Read the model definition and answer for the solid it produces. Units are mm, in the model's axes. Coordinates: 2 decimals unless noted, no trailing zeros. Order: outer loops, then holes, each group sorted by start corner. A loop starts at its lowest first (then second) coordinate and runs counter-clockwise, first axis right, second up.
```python
from build123d import *

# Parameters (mm, degrees)
SKETCH_W   = 80
SKETCH_H   = 120
SKETCH_R   = 4.5
SKETCH_R_2 = 11
SKETCH_R_3 = 3
PAD_DEPTH  = 10


with BuildPart() as part:
    # Sketch → Pad (new body)
    with BuildSketch(Plane.XY):
        with Locations((15, -15)):
            Rectangle(SKETCH_W, SKETCH_H)
        Circle(SKETCH_R, mode=Mode.SUBTRACT)
        with Locations((0, -30)):
            Circle(SKETCH_R_2, mode=Mode.SUBTRACT)
        with Locations((-10, -52)):
            Circle(SKETCH_R_3, mode=Mode.SUBTRACT)
        with Locations((40, -52)):
            Circle(SKETCH_R_3, mode=Mode.SUBTRACT)
        with Locations((40, 22)):
            Circle(SKETCH_R_3, mode=Mode.SUBTRACT)
        with Locations((-10, 22)):
            Circle(SKETCH_R_3, mode=Mode.SUBTRACT)
    extrude(amount=PAD_DEPTH)


solid = part.part
```
1) A cutting plane is placed at B-B, the plane y = -52. Determine the outline of the cut face in (x, z).
A:
outline: (-25, 0) - (-13, 0) - (-13, 10) - (-25, 10) - close; (-7, 0) - (37, 0) - (37, 10) - (-7, 10) - close; (43, 0) - (55, 0) - (55, 10) - (43, 10) - close
2) A cutting plane is placed at C-C, the plane z = 5. Determine the outline of the cut face in (x, y).
A:
outline: (-25, -75) - (55, -75) - (55, 45) - (-25, 45) - close; hole circle Ø6 at (-10, -52); hole circle Ø6 at (-10, 22); hole circle Ø22 at (0, -30); hole circle Ø9 at (0, 0); hole circle Ø6 at (40, -52); hole circle Ø6 at (40, 22)
3) A flat-ended cylindrical pin translates along its axis: pin 1 Ø2 at (x, y) = (24, -62.5) entering from -Z. Find the tip coordinate at first contact, or state that the pin passes through.
A:
pin 1: stops at z = 0
4) Straight lines are drawn through the part: line 1 (Y direction, x = 0, z = 7.5); line 2 (Y direction, x = 40, z = 9.75); line 3 (Y direction, x = -10, z = 6). For each, find the intervals that lie inside material, in ascending order.
A:
line 1: y = -75 to -41, -19 to -4.5, 4.5 to 45
line 2: y = -75 to -55, -49 to 19, 25 to 45
line 3: y = -75 to -55, -49 to -34.58, -25.42 to 19, 25 to 45
5) Determine the mould class of faces 1 (the flat face through (14, -75, 5)), 2 (the flat face through (14, -14, 10)), 3 (the cylindrical face through (-10, -49, 5)) for opening direction Y: pulls with the +Y half, pulls with the -Y half, needs draft (parallel to the pull), parting line crosses it, or undercut.
A:
face 1: pulls with the -Y half
face 2: needs draft
face 3: undercut
6) A cutting plane is placed at A-A, the plane y = 0. Determine the outline of the cut face in (x, z).
A:
outline: (-25, 0) - (-4.5, 0) - (-4.5, 10) - (-25, 10) - close; (4.5, 0) - (55, 0) - (55, 10) - (4.5, 10) - close
7) A cutting plane is placed at D-D, the plane x = 0. Determine the outline of the cut face in (y, z), and give its area (3 significant figures).
A:
outline: (-75, 0) - (-41, 0) - (-41, 10) - (-75, 10) - close; (-19, 0) - (-4.5, 0) - (-4.5, 10) - (-19, 10) - close; (4.5, 0) - (45, 0) - (45, 10) - (4.5, 10) - close
area: 890 mm2
